Input: part model. Units: mm. Frame: model coordinates. A direction names the side the tool comes from. Round coordinates to 2 decimals unless told otherwise and drop trailing zeros. Loops run counter-clockwise (first coordinate to the right, second up) from the corner with the lowest first, then second, coordinate; pieces in that order, holes last. Notation, with made-up numbers: (67, -29.5) - (74, -29.5) arc R26 cw to (74, 4.5) - close; hole circle Ø7 at (58, 69.25). An arc over 180 degrees is marked (long way). One line per question, with ' | ' between items. Start each with the question number.
Item 1: Set-up query: faces 5 (the face through (-149.97, -44.47, 82.62)), 6 (the face through (-145.9, -46.21, 81.37)), 7 (the face through (-2, 1, 5)), 8 (the face through (155, -2, 110)). Return all of +Z, -Z, +X, -X, +Y, -Y with unobstructed straight access to the full face (end or side cutting, diameter ignored); none if empty.
Item 2: Draft query along X for faces 1 (the face through (155, -2, 35)), 2 (the face through (-0.7, 108.4, 145)), 3 (the face through (-154.14, -45.24, 83.08)), 4 (the face through (-132, -91, 140)). Return one class per face: pulls with the +X half, pulls with the -X half, needs draft (parallel to the pull), parting line crosses it, or undercut.
Item 3: Section B-B, the plane z = 103.5. Return loops of the section in (x, y).
Item 4: First-contact query: pin 1 (13.5 mm diameter, centred on x = -134.5, y = 96.5, fed in from +Z); pin 2 (4 mm diameter, centred on x = 70, y = 29, fed in from +Z); pin 3 (1.5 mm diameter, centred on x = -135, z = 71.5, fed in from +Y). Flat tips, straight axial feed; report the tip coordinate or a pass-through.
Item 5: Material intervals for line 1 along Y through (x, z) = (-138, 31.5); line 2 along Y through (x, z) = (-95, 121); line 3 along X through (y, z) = (-67.5, 46), sorted ascending.
Item 6: Section A-A, the plane x = -26. Give the number of separate pieces and of enclosed holes in the cut face, plus the area to 3 significant figures.
```python
from build123d import *

# Parameters (mm, degrees)
F0_W      = 310
F0_H      = 230
F2_DEPTH  = 145
F1_W      = 290
F1_H      = 210
F3_DEPTH  = 5
F4_W      = 289.9999934435
F4_H      = 209.9999934435
F5_DEPTH  = 140
F7_DEPTH  = 310.001
F9_START  = 15
F8_W      = 30
F8_H      = 30
F9_DEPTH  = 120
F10_W     = 30
F10_H     = 209.9999934435
F11_DEPTH = 15
F12_R     = 3


with BuildPart() as f2:
    # F0 (on Top) → F2 (new body)
    with BuildSketch(Plane.XY):
        Rectangle(F0_W, F0_H)
    extrude(amount=F2_DEPTH)

    # F1 (on face) → F3 (join)
    with BuildSketch(Plane.XY):
        Rectangle(F1_W, F1_H)
    extrude(amount=-F3_DEPTH)

    # F4 (on face) → F5 (cut)
    with BuildSketch(Plane.XY.offset(145)):
        Rectangle(F4_W, F4_H)
    extrude(amount=-F5_DEPTH, mode=Mode.SUBTRACT)

    # F6 (on face) → F7 (cut, through all)
    with BuildSketch(Plane.YZ.offset(155)):
        with BuildLine():
            Line((-49, 75), (-115, 75))
            Line((-115, 75), (-115, 70))
            Line((-115, 70), (115, 70))
            Line((115, 70), (115, 75))
            Line((115, 75), (49, 75))
            Line((49, 75), (40.9071192856, 88.6107539288))
            ThreePointArc((40.9071192856, 88.6107539288), (37.256073336, 92.1921671431), (32.3117604054, 93.5))
            Line((32.3117604054, 93.5), (-32.3117604054, 93.5))
            ThreePointArc((-32.3117604054, 93.5), (-37.256073336, 92.1921671431), (-40.9071192856, 88.6107539288))
            Line((-40.9071192856, 88.6107539288), (-49, 75))
        make_face()
    extrude(amount=-F7_DEPTH, mode=Mode.SUBTRACT)

    # F8 (on face) → F9 (join)
    with BuildSketch(Plane.XY.offset(5).offset(F9_START)):
        with Locations((-129.9999967217, 89.9999967217)):
            Rectangle(F8_W, F8_H)
        with Locations((129.9999967217, 89.9999967217)):
            Rectangle(F8_W, F8_H)
        with Locations((129.9999967217, -89.9999967217)):
            Rectangle(F8_W, F8_H)
        with Locations((-129.9999967217, -89.9999967217)):
            Rectangle(F8_W, F8_H)
    extrude(amount=F9_DEPTH)

    # F10 (on face) → F11 (join)
    with BuildSketch(Plane.XY.offset(5)):
        Polygon((114.9999967217, -74.9999967217), (114.9999967217, -104.9999967217), (144.9999967217, -104.9999967217), (144.9999967217, 104.9999967217), (114.9999967217, 104.9999967217), align=None)
        with Locations((-129.9999967217, 0)):
            Rectangle(F10_W, F10_H)
    extrude(amount=F11_DEPTH)

    # F12
    f12_edges = [f2.edges().sort_by_distance(p)[0] for p in [
        (155, 0, 0),
        (155, 115, 35),
        (155, 0, 70),
        (155, -115, 35),
        (155, -82, 75),
        (155, -44.95356, 81.805377),
        (155, -37.256073, 92.192167),
        (155, 0, 93.5),
        (155, 37.256073, 92.192167),
        (155, 44.95356, 81.805377),
        (155, 82, 75),
        (155, 115, 110),
        (155, 0, 145),
        (155, -115, 110),
        (0, -115, 0),
        (0, -115, 70),
        (-155, -115, 35),
        (0, -115, 75),
        (0, -115, 145),
        (-155, -115, 110),
        (-155, 82, 75),
        (-155, 44.95356, 81.805377),
        (-155, 37.256073, 92.192167),
        (-155, 0, 93.5),
        (-155, -37.256073, 92.192167),
        (-155, -44.95356, 81.805377),
        (-155, -82, 75),
        (-155, 0, 145),
        (-155, 115, 110),
        (-155, 0, 0),
        (-155, 0, 70),
        (-155, 115, 35),
        (0, 115, 0),
        (0, 115, 70),
        (0, 115, 75),
        (0, 115, 145),
        (0, 104.999997, 145),
        (144.999997, 0, 145),
        (0, -104.999997, 145),
        (-144.999997, 0, 145),
        (-129.999997, -74.999997, 140),
        (-114.999997, -89.999997, 140),
        (-114.999997, -74.999997, 80),
        (114.999997, -89.999997, 140),
        (114.999997, -74.999997, 80),
        (129.999997, -74.999997, 140),
        (114.999997, 0, 20),
        (114.999997, 74.999997, 80),
        (129.999997, 74.999997, 140),
        (-114.999997, 0, 20),
        (-114.999997, 74.999997, 80),
        (-129.999997, 74.999997, 140),
        (144.999997, 0, 70),
        (-144.999997, 0, 70),
        (-144.999997, 37.256073, 92.192167),
        (144.999997, 37.256073, 92.192167),
        (149.999998, -49, 75),
        (149.999998, 49, 75),
        (0, 105, -5),
        (-145, 0, -5),
        (0, -105, -5),
        (145, 0, -5),
        (-149.999998, -49, 75),
        (-149.999998, 49, 75),
        (144.999997, 44.95356, 81.805377),
        (144.999997, 0, 93.5),
        (144.999997, -37.256073, 92.192167),
        (144.999997, -44.95356, 81.805377),
        (-144.999997, -44.95356, 81.805377),
        (-144.999997, -37.256073, 92.192167),
        (-144.999997, 0, 93.5),
        (-144.999997, 44.95356, 81.805377),
    ]]
    fillet(f12_edges, radius=F12_R)


solid = f2.part
```
Return value:
1) face 5: +X, -X | face 6: none | face 7: +Z | face 8: +Z, -Z, +X, +Y, -Y
2) face 1: pulls with the +X half | face 2: needs draft | face 3: pulls with the -X half | face 4: undercut
3) outline: (-155, -112) arc R3 ccw to (-152, -115) - (152, -115) arc R3 ccw to (155, -112) - (155, 112) arc R3 ccw to (152, 115) - (-152, 115) arc R3 ccw to (-155, 112) - close; hole (-145, -75) - (-118, -75) arc R3 cw to (-115, -78) - (-115, -105) - (115, -105) - (115, -78) arc R3 cw to (118, -75) - (145, -75) - (145, 75) - (118, 75) arc R3 cw to (115, 78) - (115, 105) - (-115, 105) - (-115, 78) arc R3 cw to (-118, 75) - (-145, 75) - close
4) pin 1: z = 140 | pin 2: z = 5 | pin 3: y = 105
5) line 1: -115 to -75, 75 to 115 | line 2: -115 to -105, 105 to 115 | line 3: -155 to -145, 145 to 155
6) separate pieces: 3 | enclosed holes: 0 | area: 4,880 mm2
